Geometry: final body of the model. Coordinates: model frame, mm. Face numbers are marked on the shaded views. A direction names the side the tool comes from. Give positions to 0.01 mm unless a question says otherwise; leave off trailing zeros. Write each loop counter-clockwise with the first axis right and the second up, starting at its lowest first coordinate (ties: lowest second). Pieces come first, ordered by that corner, then holes. Notation, with made-up numbers: M 40,38 L 77,38 A19 ccw 77,69 Z; hole C 17.25,4.25 d8. An arc over 180 degrees is marked long. Use a Markdown table: item, result. Add a question column.
(1) Cut plane D-D (x = -26). Output: boundary loops of the cut face in (y, z).
(2) Material intervals for L1, parallel to Z at x = 39, y = 2; L2, parallel to X at y = 3, z = -24; L3, parallel to X at y = 17, z = -35.5, sorted ascending.
(3) Pin query (flat end, axial travel): pin 1 Ø9.5 at (x, z) = (57.5, -75.5) entering from +Y; pin 2 Ø1.3 at (x, y) = (-18, 14.5) entering from -Z; pin 3 Ø10 at (x, z) = (41, -1) entering from +Y; pin 4 Ø10 at (x, y) = (20, 3.5) entering from +Z. Return the tip coordinate at first contact, or that it passes through.
(4) Reachability of the marked faces 1, 2 and 3 from +Z, -Z, +X, -X, +Y, -Y: full face, straight path, thin tool, end or side. Return the list, or none.
(5) Cut plane B-B (x = 3). Output: boundary loops of the cut face in (y, z).
(6) Cut plane A-A (y = 15.5). Output: boundary loops of the cut face in (x, z), plus the area to 3 significant figures.
(7) Cut plane C-C (z = -24). Output: boundary loops of the cut face in (x, y), plus the area to 3 significant figures.
```python
from build123d import *

# Parameters (mm, degrees)
BOSS_EXTRUDE1_DEPTH  = 19.05
BOSS_EXTRUDE2_DEPTH  = 19.05
BOSS_EXTRUDE3_DEPTH  = 19.05
BOSS_EXTRUDE4_DEPTH  = 19.05
BOSS_EXTRUDE13_DEPTH = 19.05
CUT_EXTRUDE1_REACH   = 84.55
SKETCH14_R           = 1.778
SKETCH14_W           = 3.048
SKETCH14_H           = 3.81


with BuildPart() as part:
    # Sketch1 → Boss-Extrude1 (new body)
    with BuildSketch(Plane.XY):
        Polygon((0, 0), (44.45, 2.329525789), (63.5, 2.329525789), (63.5, 0), align=None)
    extrude(amount=BOSS_EXTRUDE1_DEPTH)

    # Sketch2 → Boss-Extrude2 (add)
    with BuildSketch(Plane(origin=(63.5, 0, 0), x_dir=(0, 0, -1), z_dir=(1, 0, 0))):
        Polygon((0, 0), (0, 2.329525789), (63.5, 5.657419774), (82.55, 5.657419774), (82.55, 0), align=None)
    extrude(amount=-BOSS_EXTRUDE2_DEPTH)

    # Sketch3 → Boss-Extrude3 (add)
    with BuildSketch(Plane(origin=(0, 0, -82.55), x_dir=(-1, 0, 0), z_dir=(0, 0, -1))):
        Polygon((-44.45, 0), (-44.45, 5.657419774), (19.05, 8.985313758), (38.1, 8.985313758), (38.1, 0), align=None)
    extrude(amount=-BOSS_EXTRUDE3_DEPTH)

    # Sketch4 → Boss-Extrude4 (add)
    with BuildSketch(Plane.ZY.offset(38.1)):
        Polygon((-63.5, 8.985313758), (-38.1, 10.316471352), (-19.05, 10.316471352), (-19.05, 0), (-63.5, 0), align=None)
    extrude(amount=-BOSS_EXTRUDE4_DEPTH)

    # Sketch13 → Boss-Extrude13 (add)
    with BuildSketch(Plane.XY.offset(-19.05)):
        Polygon((-19.05, 5.917062301), (-19.05, 23.016471352), (-16.51, 23.016471352), (-16.51, 10.316471352), align=None)
    extrude(amount=-BOSS_EXTRUDE13_DEPTH)

    # Sketch14 → Cut-Extrude1 (cut, up to next)
    with BuildSketch(Plane.ZY.offset(19.05), mode=Mode.PRIVATE) as cut_extrude1_sk1:
        with Locations((-28.575, 20.222471352)):
            Circle(SKETCH14_R)
    cut_extrude1_tool1 = extrude(cut_extrude1_sk1.sketch, amount=-CUT_EXTRUDE1_REACH, mode=Mode.PRIVATE) & part.part
    add(cut_extrude1_tool1.solids().sort_by_distance((-19.05, 20.222471, -28.575))[0], mode=Mode.SUBTRACT)
    # Sketch14 → Cut-Extrude1 (cut, up to next)
    with BuildSketch(Plane.ZY.offset(19.05), mode=Mode.PRIVATE) as cut_extrude1_sk2:
        with Locations((-28.575, 15.269471352)):
            Rectangle(SKETCH14_W, SKETCH14_H)
    cut_extrude1_tool2 = extrude(cut_extrude1_sk2.sketch, amount=-CUT_EXTRUDE1_REACH, mode=Mode.PRIVATE) & part.part
    add(cut_extrude1_tool2.solids().sort_by_distance((-19.05, 15.269471, -28.575))[0], mode=Mode.SUBTRACT)


solid = part.part
```
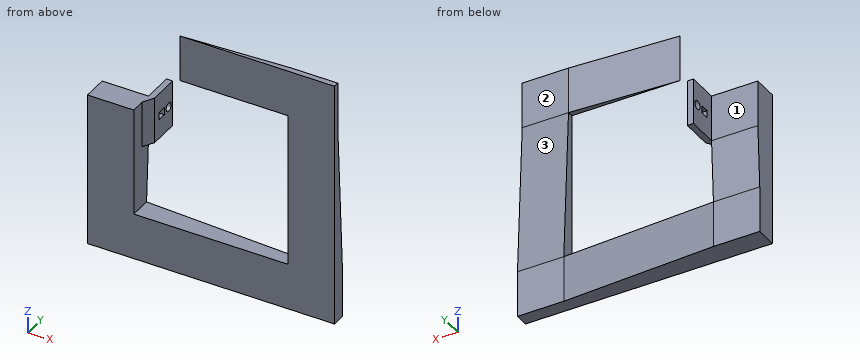
Answer list:
| question | item | result |
|---|---|---|
| 1 | outline | M 0,-82.55 L 8.99,-82.55 L 8.99,-63.5 L 10.32,-38.1 L 10.32,-19.05 L 0,-19.05 Z |
| 2 | L1 | -82.55 to -63.5, 0 to 19.05 |
| 2 | L2 | -38.1 to -19.05, 44.45 to 63.5 |
| 2 | L3 | -19.05 to -16.51 |
| 3 | pin 1 | y = 5.66 |
| 3 | pin 2 | z = -38.1 |
| 3 | pin 3 | y = 2.57 |
| 3 | pin 4 | z = 19.05 |
| 4 | face 1 | +Z, -Z, -X, +Y |
| 4 | face 2 | +Z, +X, -X, +Y |
| 4 | face 3 | +Z, +X, +Y |
| 5 | outline | M 0,-82.55 L 7.83,-82.55 L 7.83,-63.5 L 0,-63.5 Z; M 0,0 L 0.16,0 L 0.16,19.05 L 0,19.05 Z |
| 6 | outline | M -19.05,-38.1 L -16.51,-38.1 L -16.51,-30.1 L -19.05,-30.1 Z; M -19.05,-27.05 L -16.51,-27.05 L -16.51,-19.05 L -19.05,-19.05 Z |
| 6 | area | 40.6 mm² |
| 7 | outline | M -38.1,0 L -19.05,0 L -19.05,5.92 L -16.51,10.32 L -16.51,23.02 L -19.05,23.02 L -19.05,10.32 L -38.1,10.32 Z; M 44.45,0 L 63.5,0 L 63.5,3.59 L 44.45,3.59 Z |
| 7 | area | 303 mm² |
